Source: CAD feature listing. Evaluate the final solid. Frame: model axes, mm. Face numbers are marked on the shaded views. A direction names the side the tool comes from. Give positions to 0.01 mm unless a question says otherwise; leave off trailing zeros. Order: outer loops, then holes, each group sorted by start corner. A loop starts at its lowest first (then second) coordinate and runs counter-clockwise, first axis right, second up. Notation, with made-up numbers: M 41,-15.75 L 55,-15.75 A18 cw 55,7.25 Z; hole C 70,85 d10. An arc over 180 degrees is marked long. Use CSV: the item, a comma, the result in double quotes. Start each with the question number.
Item 1: Section query D-D on x = 1. Return loops of the section in (y, z).
Item 2: Section query C-C on z = 0. Return loops of the section in (x, y).
Item 3: Ray query, probe 1 along X at (y, z) = (-2, -11.5); probe 2 along Z at (x, y) = (0, -3); probe 3 along Z at (x, y) = (8, -5). Return the intervals inside material, ascending. Write a range as from..to.
Item 4: Access query for the marked faces 4, 5 and 6. Directions: +Z, -Z, +X, -X, +Y, -Y. A direction counts if a zero-diameter tool reaches every point of the face in a straight line with its end or side. Return the directions, or none.
Item 5: First-contact query: pin 1 (1.5 mm diameter, centred on y = -4, z = -13.5, fed in from +X); pin 2 (1.5 mm diameter, centred on y = -5, z = 35.5, fed in from -X); pin 3 (2 mm diameter, centred on x = 12, y = -3, fed in from -Z). Flat tips, straight axial feed; report the tip coordinate or a pass-through.
Item 6: Pull-direction query (Z, two-part tool) for the marked faces 1, 2 and 3; classes: +Z half, -Z half, draft (parallel to the pull), parting line (faces both ways), or undercut.
Item 7: Section query B-B on x = 22.5. Return loops of the section in (y, z).
Item 8: Section query A-A on y = -3.5. Count the separate pieces of the cut face and the enclosed holes in it, and give its area (3 significant figures).
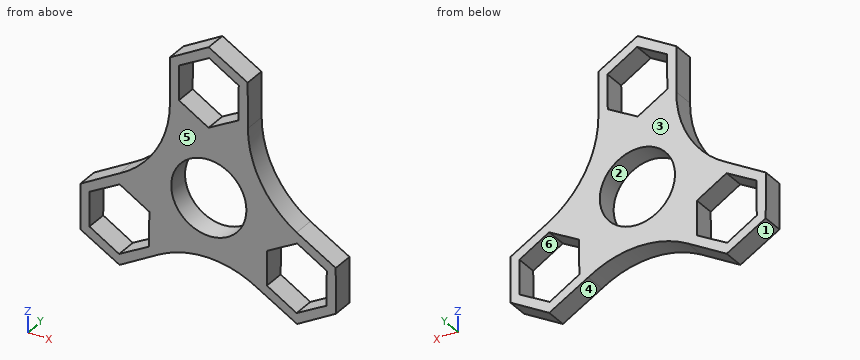
from build123d import *

# Parameters (mm, degrees)
F0_R     = 14.2875
F0_R_2   = 11.0236
F1_DEPTH = 6.35


# Not quite as in the source:
# - a feature names something its author has since deleted; it is built from what else it names


with BuildPart() as f1:
    # F0 (on Front) → F1 (new body)
    with BuildSketch(Plane.XZ):
        with BuildLine():
            ThreePointArc((25.7649177957, -1.6892582355), (15.3069411381, 9.1784817197), (11.4569144183, 23.7611543748))
            Line((11.4569144183, 23.7611543748), (0.05402032, 17.115313105))
            Line((0.05402032, 17.115313105), (-11.4028940983, 23.6675884359))
            ThreePointArc((-11.4028940983, 23.6675884359), (-15.3765179084, 9.0528933251), (-26.2895962669, -1.4487122715))
            Line((-26.2895962669, -1.4487122715), (-14.8326818486, -8.0009876024))
            Line((-14.8326818486, -8.0009876024), (-14.7786615286, -21.1991042031))
            ThreePointArc((-14.7786615286, -21.1991042031), (-0.135152389, -17.3330158123), (14.4160440174, -21.533216106))
            Line((14.4160440174, -21.533216106), (14.3620236974, -8.3350995053))
            Line((14.3620236974, -8.3350995053), (25.7649177957, -1.6892582355))
        make_face()
        Circle(F0_R, mode=Mode.SUBTRACT)
        Circle(F0_R)
        Circle(F0_R_2, mode=Mode.SUBTRACT)
        Polygon((11.4028940983, 36.9592709755), (-0.05402032, 43.5115463064), (-11.4569144183, 36.8657050366), (-11.4028940983, 23.6675884359), (0.05402032, 17.115313105), (11.4569144183, 23.7611543748), align=None)
        Polygon((-8.6923295278, 35.4356960394), (0.089848006, 40.4023410617), (8.7821775338, 35.280074728), (8.6923295278, 25.191163372), (-0.089848006, 20.2245183497), (-8.7821775338, 25.3467846834), align=None, mode=Mode.SUBTRACT)
        Polygon((37.221832214, -8.2415335664), (25.7649177957, -1.6892582355), (14.3620236974, -8.3350995053), (14.4160440174, -21.533216106), (25.8729584357, -28.0854914369), (37.275852534, -21.4396501671), align=None)
        Polygon((17.1266085879, -9.7651085025), (25.9087861217, -4.7984634802), (34.6011156495, -9.9207298139), (34.5112676435, -20.0096411699), (25.7290901097, -24.9762861922), (17.0367605819, -19.8540198585), align=None, mode=Mode.SUBTRACT)
        Polygon((-14.8326818486, -8.0009876024), (-26.2895962669, -1.4487122715), (-37.6924903652, -8.0945535413), (-37.6384700452, -21.292670142), (-26.1815556269, -27.8449454729), (-14.7786615286, -21.1991042031), align=None)
        Polygon((-17.4533984131, -9.6801838499), (-17.5432464191, -19.7690952059), (-26.325423953, -24.7357402282), (-35.0177534808, -19.6134738945), (-34.9279054747, -9.5245625385), (-26.1457279409, -4.5579175162), align=None, mode=Mode.SUBTRACT)
    extrude(amount=F1_DEPTH)


solid = f1.part
Verdict:
1,outline,"M -6.35,-17.37 L 0,-17.37 L 0,-10.98 L -6.35,-10.98 Z; M -6.35,10.98 L 0,10.98 L 0,20.84 L -6.35,20.84 Z; M -6.35,39.87 L 0,39.87 L 0,42.91 L -6.35,42.91 Z"
2,outline,"M -23.9,-6.35 L -11.02,-6.35 L -11.02,0 L -23.9,0 Z; M 11.02,-6.35 L 23.3,-6.35 L 23.3,0 L 11.02,0 Z"
3,probe 1,"-37.68..-34.95, -17.47..17.11, 34.59..37.24"
3,probe 2,"-17.33..-11.02, 11.02..20.28, 40.35..43.48"
3,probe 3,"-18.62..-7.58, 7.58..24.8, 35.74..38.91"
4,face 4,"-Z, +Y, -Y"
4,face 5,"+Z, -Z, +X, -X, -Y"
4,face 6,"+Y, -Y"
5,pin 1,"x = 37.25"
5,pin 2,"x = -11.45"
5,pin 3,"z = -20.72"
6,face 1,"-Z half"
6,face 2,"undercut"
6,face 3,"draft"
7,outline,"M -6.35,-26.16 L 0,-26.16 L 0,-23.07 L -6.35,-23.07 Z; M -6.35,-6.73 L 0,-6.73 L 0,0.63 L -6.35,0.63 Z"
8,separate pieces,"1"
8,enclosed holes,"4"
8,area,"1,470 mm2"
